```python
from build123d import *

# Parameters (mm, degrees)
SKETCH1_R               = 4
BOSS_EXTRUDE1_DEPTH     = 12.5
SKETCH2_W               = 60
SKETCH2_H               = 10
BOSS_EXTRUDE2_DEPTH     = 15
CHAMFER1_SIZE           = 2
SKETCH3_R               = 2.25
CUT_EXTRUDE1_DEPTH      = 45.5
CUT_EXTRUDE2_REACH      = 51.399
CUT_EXTRUDE2_END_RADIUS = 4
SKETCH4_R               = 1.25


with BuildPart() as part:
    # Sketch1 → Boss-Extrude1 (new, symmetric)
    with BuildSketch(Plane(origin=(0, 0, 0), x_dir=(1, 0, 0), z_dir=(0, 1, 0))):
        Polygon((-15, -9), (-30, -9), (-30, -19), (30, -19), (30, -9), (15, -9), (15, 9), (-15, 9), align=None)
        with Locations(Location((0, 0, 0), (0, 0, 270))):
            Circle(SKETCH1_R, mode=Mode.SUBTRACT)
    extrude(amount=BOSS_EXTRUDE1_DEPTH, both=True)

    # Sketch2 → Boss-Extrude2 (add)
    with BuildSketch(Plane(origin=(0, 12.5, 0), x_dir=(1, 0, 0), z_dir=(0, 1, 0))):
        with Locations((0, -14)):
            Rectangle(SKETCH2_W, SKETCH2_H)
    extrude(amount=BOSS_EXTRUDE2_DEPTH)

    # Chamfer1
    chamfer1_edges = [part.edges().sort_by_distance(p)[0] for p in [
        (30, 7.5, 19),
        (-30, 7.5, 19),
        (-30, 27.5, 14),
        (0, 27.5, 19),
        (30, 27.5, 14),
    ]]
    chamfer(chamfer1_edges, length=CHAMFER1_SIZE)

    # Sketch3 → Cut-Extrude1 (cut, through all)
    with BuildSketch(Plane(origin=(0, 0, 9), x_dir=(-1, 0, 0), z_dir=(0, 0, -1))):
        with Locations((-22.5, 20.5)):
            Circle(SKETCH3_R)
        with Locations((-22.5, -4.5)):
            Circle(SKETCH3_R)
        with Locations((22.5, 20.5)):
            Circle(SKETCH3_R)
        with Locations((22.5, -4.5)):
            Circle(SKETCH3_R)
    extrude(amount=-CUT_EXTRUDE1_DEPTH, mode=Mode.SUBTRACT)

    # Cut-Extrude2: up to this cylinder (the profile starts outside it)
    cut_extrude2_end = Plane(origin=(0, -0.5, 0), z_dir=(0, -1, 0)) * Cylinder(CUT_EXTRUDE2_END_RADIUS, 111.798, mode=Mode.PRIVATE)
    # Sketch4 → Cut-Extrude2 (cut, up to the surface)
    with BuildSketch(Plane.XY.offset(19), mode=Mode.PRIVATE) as cut_extrude2_sk1:
        with Locations((0, -0.5)):
            Circle(SKETCH4_R)
    cut_extrude2_tool1 = extrude(cut_extrude2_sk1.sketch, amount=-CUT_EXTRUDE2_REACH, mode=Mode.PRIVATE) - cut_extrude2_end
    add(cut_extrude2_tool1.solids().sort_by_distance((0, -0.5, 19))[0], mode=Mode.SUBTRACT)


solid = part.part
```
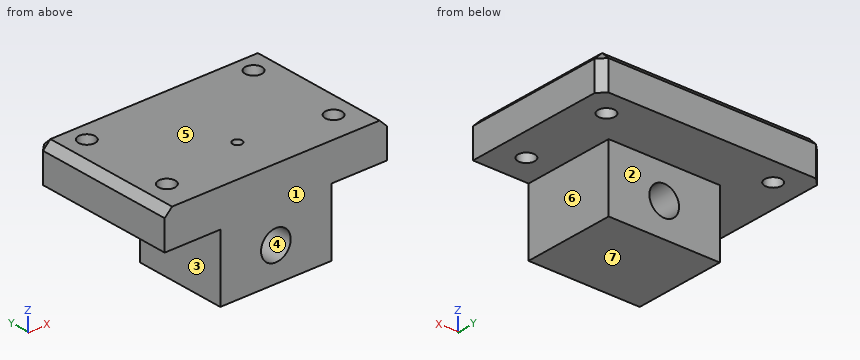
Work out the finished part from the listing and answer in its coordinate system (mm). Face numbers are marked on the shaded views. A direction names the side the tool comes from. Give positions to 0.01 mm unless a question says otherwise; leave off trailing zeros. Loops run counter-clockwise (first coordinate to the right, second up) from the corner with the lowest first, then second, coordinate; pieces in that order, holes last. Notation, with made-up numbers: (60, 10.5) -> (87, 10.5) arc R11 cw to (87, 14.5) -> close; hole circle Ø1 at (60, -9). An arc over 180 degrees is marked (long way). One line per question, with ' | ' between items. Start each with the question number.
1) Section A-A, the plane y = 20.5 is taken. Determine the outline of the cut face in (x, z), then the cut area to 3 significant figures.
2) For the marked faces 1, 2 and 3, determine the directions among +Z, -Z, +X, -X, +Y, -Y from which every point of the face is accessible in a straight line to the end or side of a thin tool.
3) Section D-D, the plane y = 5 is taken. Determine the outline of the cut face in (x, z), then the cut area to 3 significant figures.
4) Section C-C, the plane x = 22.5 is taken. Determine the outline of the cut face in (y, z), then the cut area to 3 significant figures.
5) Section B-B, the plane z = 0 is taken. Determine the outline of the cut face in (x, y).
6) Straight lines are drawn through the part: L1, parallel to Y at x = 0, z = 10.5; L2, parallel to Y at x = 21, z = 16.5; L3, parallel to X at y = -7.5, z = 0. For each, find the intervals that lie inside material, in ascending order.
7) Each of these flat-tipped pins is pushed along its axis until it touches: pin 1 (10 mm diameter, centred on x = 14.5, z = 1.5, fed in from +Y); pin 2 (7 mm diameter, centred on x = 22.5, y = 20.5, fed in from -Z); pin 3 (12 mm diameter, centred on y = 8.5, z = 0, fed in from +X). Where does it stop, or does it pass through?
8) Determine the mould class of the marked faces 4, 5, 6 and 7 for opening direction Z: +Z half, -Z half, draft (parallel to the pull), parting line (faces both ways), or undercut.
Resolved:
1) outline: (-30, 9) -> (-24.75, 9) -> (-24.75, 19) -> (-28, 19) -> (-30, 17) -> close; (-20.25, 9) -> (20.25, 9) -> (20.25, 19) -> (-20.25, 19) -> close; (24.75, 9) -> (30, 9) -> (30, 17) -> (28, 19) -> (24.75, 19) -> close | area: 506 mm2
2) face 1: +Z, -Z, +X, -X, -Y | face 2: -Z, +X, -X, +Y | face 3: -Z, -X, +Y, -Y
3) outline: (-30, 9) -> (-15, 9) -> (-15, -9) -> (15, -9) -> (15, 9) -> (30, 9) -> (30, 17) -> (28, 19) -> (-28, 19) -> (-30, 17) -> close; hole circle Ø8 at (0, 0) | area: 1,090 mm2
4) outline: (-12.5, 9) -> (-6.75, 9) -> (-6.75, 19) -> (-12.5, 19) -> close; (-2.25, 9) -> (18.25, 9) -> (18.25, 19) -> (-2.25, 19) -> close; (22.75, 9) -> (27.5, 9) -> (27.5, 17) -> (25.5, 19) -> (22.75, 19) -> close | area: 308 mm2
5) outline: (-15, -12.5) -> (-4, -12.5) -> (-4, 12.5) -> (-15, 12.5) -> close; (4, -12.5) -> (15, -12.5) -> (15, 12.5) -> (4, 12.5) -> close
6) L1: -12.5 to -1.75, 0.75 to 27.5 | L2: -12.5 to -6.18, -2.82 to 18.82, 22.18 to 27.5 | L3: -15 to -4, 4 to 15
7) pin 1: y = 12.5 | pin 2: z = 9 | pin 3: x = 15
8) face 4: undercut | face 5: +Z half | face 6: draft | face 7: -Z half
